Geometry check sheet. Reference: the model listing, model coordinates, mm. Face numbers are marked on the shaded views. Coordinates: 2 decimals unless noted, no trailing zeros. Order: outer loops, then holes, each group sorted by start corner. A loop starts at its lowest first (then second) coordinate and runs counter-clockwise, first axis right, second up. Notation, with made-up numbers: (48.5, -10) -> (92.5, -10) arc R11 ccw to (92.5, 10) -> close; hole circle Ø10 at (77.5, -18.75). An arc over 180 degrees is marked (long way). Answer as CSV lines item,"result". Start each with the question number.
from build123d import *

# Parameters (mm, degrees)
F0_W     = 50
F0_H     = 50
F1_DEPTH = 20
F2_R     = 10
F3_DEPTH = 20.001
F4_R     = 2


with BuildPart() as f1:
    # F0 (on Top) → F1 (new body)
    with BuildSketch(Plane.XY):
        Rectangle(F0_W, F0_H)
    extrude(amount=F1_DEPTH)

    # F2 (on face) → F3 (cut, through all)
    with BuildSketch(Plane.XY.offset(20)):
        Circle(F2_R)
    extrude(amount=-F3_DEPTH, mode=Mode.SUBTRACT)

    # F4
    f4_edges = [f1.edges().sort_by_distance(p)[0] for p in [
        (-25, -25, 10),
        (25, -25, 10),
        (-25, 25, 10),
        (25, 25, 10),
    ]]
    fillet(f4_edges, radius=F4_R)


solid = f1.part
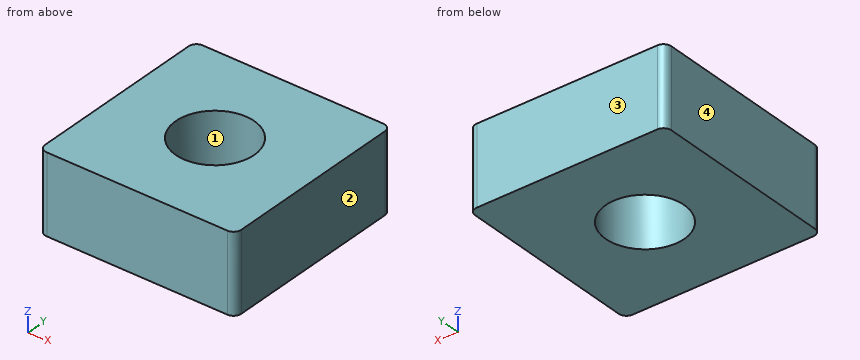
Q1. Sectioned sample at A-A, the plane x = 0. Record the cut outline in (y, z).
Q2. Sectioned sample at C-C, the plane z = 17.5. Record the cut outline in (x, y).
Q3. Release check for a two-part mould opening along X. For the marked faces 1, 2, 3 and 4 record: released by +X, released by -X, zero draft, split by the parting line, or undercut.
Q4. Thickness scan on L1, parallel to Y at x = 0, z = 8.5; L2, parallel to X at y = 4, z = 5; L3, parallel to X at y = -9, z = 3.75. Record the ranges inside material, lowest first.
Geometry results:
1,outline,"(-25, 0) -> (-10, 0) -> (-10, 20) -> (-25, 20) -> close; (10, 0) -> (25, 0) -> (25, 20) -> (10, 20) -> close"
2,outline,"(-25, -23) arc R2 ccw to (-23, -25) -> (23, -25) arc R2 ccw to (25, -23) -> (25, 23) arc R2 ccw to (23, 25) -> (-23, 25) arc R2 ccw to (-25, 23) -> close; hole circle Ø20 at (0, 0)"
3,face 1,"undercut"
3,face 2,"released by +X"
3,face 3,"zero draft"
3,face 4,"released by -X"
4,L1,"y = -25 to -10, 10 to 25"
4,L2,"x = -25 to -9.17, 9.17 to 25"
4,L3,"x = -25 to -4.36, 4.36 to 25"
